```python
from build123d import *

# Parameters (mm, degrees)
SKETCH1_W                       = 20
SKETCH1_H                       = 20
BOSS_EXTRUDE1_DEPTH             = 30
F_3_0MM_DOWEL_HOLE1_D           = 3
F_3_0MM_DOWEL_HOLE1_DEPTH       = 20
F_3_0MM_DOWEL_HOLE1_CSINK_D     = 3.05
F_3_0MM_DOWEL_HOLE1_CSINK_ANGLE = 90
F_3_0MM_DOWEL_HOLE1_TIP         = 0.901290929
F_3_0MM_DOWEL_HOLE2_D           = 3
F_3_0MM_DOWEL_HOLE2_DEPTH       = 20
F_3_0MM_DOWEL_HOLE2_CSINK_D     = 3.05
F_3_0MM_DOWEL_HOLE2_CSINK_ANGLE = 90
F_3_0MM_DOWEL_HOLE2_TIP         = 0.901290929


with BuildPart() as part:
    # Sketch1 → Boss-Extrude1 (new body)
    with BuildSketch(Plane(origin=(0, 0, 0), x_dir=(1, 0, 0), z_dir=(0, 1, 0))):
        with Locations((10, -10)):
            Rectangle(SKETCH1_W, SKETCH1_H)
    extrude(amount=BOSS_EXTRUDE1_DEPTH)

    # Ø3.0mm Dowel Hole1
    with Locations(Plane(origin=(20, 0, 0), x_dir=(0, 0, -1), z_dir=(1, 0, 0))):
        with Locations((-10, 8)):
            CounterSinkHole(F_3_0MM_DOWEL_HOLE1_D / 2, F_3_0MM_DOWEL_HOLE1_CSINK_D / 2, depth=F_3_0MM_DOWEL_HOLE1_DEPTH, counter_sink_angle=F_3_0MM_DOWEL_HOLE1_CSINK_ANGLE)
            with Locations((0, 0, -(F_3_0MM_DOWEL_HOLE1_DEPTH + F_3_0MM_DOWEL_HOLE1_TIP / 2))):  # 118° drill point
                Cone(0, F_3_0MM_DOWEL_HOLE1_D / 2, F_3_0MM_DOWEL_HOLE1_TIP, mode=Mode.SUBTRACT)

    # Ø3.0mm Dowel Hole2
    with Locations(Plane.XY.offset(20)):
        with Locations((10, 22)):
            CounterSinkHole(F_3_0MM_DOWEL_HOLE2_D / 2, F_3_0MM_DOWEL_HOLE2_CSINK_D / 2, depth=F_3_0MM_DOWEL_HOLE2_DEPTH, counter_sink_angle=F_3_0MM_DOWEL_HOLE2_CSINK_ANGLE)
            with Locations((0, 0, -(F_3_0MM_DOWEL_HOLE2_DEPTH + F_3_0MM_DOWEL_HOLE2_TIP / 2))):  # 118° drill point
                Cone(0, F_3_0MM_DOWEL_HOLE2_D / 2, F_3_0MM_DOWEL_HOLE2_TIP, mode=Mode.SUBTRACT)


solid = part.part
```
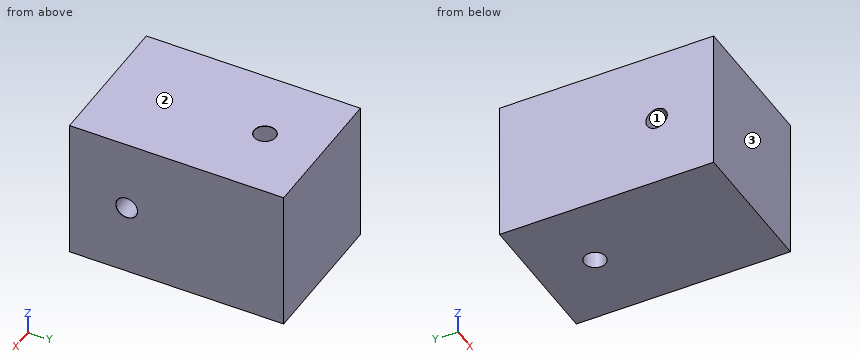
Input: part model. Units: mm. Frame: model coordinates. Face numbers are marked on the shaded views. Round coordinates to 2 decimals unless told otherwise and drop trailing zeros. Loops run counter-clockwise (first coordinate to the right, second up) from the corner with the lowest first, then second, coordinate; pieces in that order, holes last. Notation, with made-up numbers: (-3.75, 86) - (13.25, 86) arc R18 cw to (13.25, 107) - close; hole circle Ø2 at (-21, -14). An arc over 180 degrees is marked (long way). One line per item, written item: value. Start each with the question number.
(1) Section B-B, the plane y = 22. Return loops of the section in (x, z) (3 decimals).
(2) Contact query for flat-ended pins moving along their axis: P1, Ø3.5, axis at y = 8, z = 10, coming from the -X side; P2, Ø2.5, axis at x = 10, y = 22, coming from the +Z side. Output: stop coordinate, or through.
(3) Ray query, line 1 (Y direction, x = 10, z = 5.75); line 2 (Z direction, x = 10.75, y = 8). Return the intervals inside material, ascending. Write a range as [from, to].
(4) Section C-C, the plane z = 10. Return loops of the section in (x, y) (3 decimals), plus the area to 3 significant figures.
(5) Section A-A, the plane x = 10. Return loops of the section in (y, z) (3 decimals), plus the area to 3 significant figures.
(6) Draft query along Y for the marked faces 1, 2 and 3. Return one class per face: +Y half, -Y half, draft (parallel to the pull), parting line (faces both ways), or undercut.
Results below:
1. outline: (0, 0) - (8.5, 0) - (8.5, 19.975) - (8.475, 20) - (0, 20) - close; (11.5, 0) - (20, 0) - (20, 20) - (11.525, 20) - (11.5, 19.975) - close
2. P1: x = 0
2. P2: through
3. line 1: [0, 20.5], [23.5, 30]
3. line 2: [0, 8.5], [11.5, 20]
4. outline: (0, 0) - (20, 0) - (20, 6.475) - (19.975, 6.5) - (0, 6.5) - close; (0, 9.5) - (19.975, 9.5) - (20, 9.525) - (20, 30) - (0, 30) - close; hole circle Ø3 at (10, 22)
4. area: 533 mm^2
5. outline: (0, 0) - (20.5, 0) - (20.5, 19.975) - (20.475, 20) - (0, 20) - close; (23.5, 0) - (30, 0) - (30, 20) - (23.525, 20) - (23.5, 19.975) - close; hole circle Ø3 at (8, 10)
5. area: 533 mm^2
6. face 1: undercut
6. face 2: draft
6. face 3: -Y half
